Answer from the drawing. Dimensions are ordinates in mm from the lowest x, y and z of the part. A direction names the side the tool comes from. Coordinates: 2 decimals unless noted, no trailing zeros. Loops run counter-clockwise (first coordinate to the right, second up) from the corner with the lowest first, then second, coordinate; pieces in that order, holes last. Notation, with made-up numbers: M -7,-39.5 L 31,-39.5 A27 cw 31,-17.5 Z; hole C 40.25,48.5 d4. An arc over 180 degrees is marked long. Answer as CSV lines item,"result". Start each with the question number.
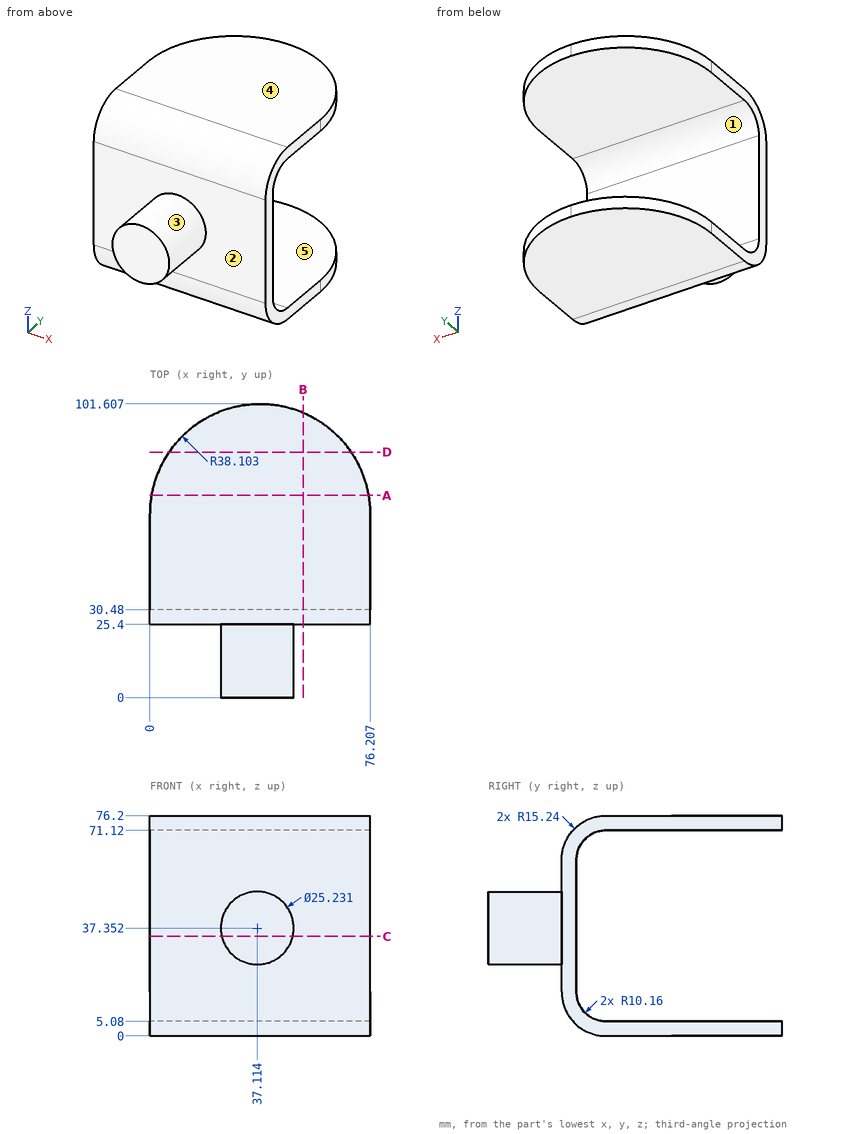
Item 1: Consider line 1 (Z direction, x = 67.5, y = 86); line 2 (Y direction, x = 31, z = 29); line 3 (Y direction, x = 37, z = 23). Determine where each line is inside the solid, lowest interval first.
Item 2: Section D-D on y = 85 is taken. Determine the outline of the cut face in (x, z) (1 decimal).
Item 3: For the marked faces 4 and 5, determine the directions among +Z, -Z, +X, -X, +Y, -Y from which every point of the face is accessible in a straight line to the end or side of a thin tool.
Item 4: Section A-A on y = 70 is taken. Determine the outline of the cut face in (x, z), then the cut area to 3 significant figures.
Item 5: Section C-C on z = 34.5 is taken. Determine the outline of the cut face in (x, y) (1 decimal).
Item 6: Section B-B on x = 53 is taken. Determine the outline of the cut face in (y, z) (1 decimal).
Item 7: Each of these flat-tipped pins is pushed along its axis until it touches: P1, Ø10, axis at x = 35, z = 52, coming from the +Y side; P2, Ø2, axis at x = 13.5, y = 24, coming from the +Z side; P3, Ø3, axis at x = 48.5, y = 37.5, coming from the -Z side; P4, Ø2, axis at x = 33, y = 10.5, coming from the +Z side. Where does it stop, or does it pass through?
Item 8: For a pull along Z with two mould halves and no side action, classify the marked faces 1, 2 and 3 as pulls with the +Z half, pulls with the -Z half, needs draft (parallel to the pull), parting line crosses it, or undercut.
Results are:
1,line 1,"0 to 5.08, 71.12 to 76.2"
1,line 2,"0 to 30.48"
1,line 3,"25.4 to 30.48"
2,outline,"M 6.6,0 L 69.6,0 L 69.6,5.1 L 6.6,5.1 Z; M 6.6,71.1 L 69.6,71.1 L 69.6,76.2 L 6.6,76.2 Z"
3,face 4,"+Z, +X, -X, +Y, -Y"
3,face 5,"+X, -X, +Y"
4,outline,"M 0.56,0 L 75.65,0 L 75.65,5.08 L 0.56,5.08 Z; M 0.56,71.12 L 75.65,71.12 L 75.65,76.2 L 0.56,76.2 Z"
4,area,"763 mm²"
5,outline,"M 0,25.4 L 24.8,25.4 L 24.8,0 L 49.4,0 L 49.4,25.4 L 76.2,25.4 L 76.2,30.5 L 0,30.5 Z"
6,outline,"M 25.4,15.2 A15.2 ccw 40.6,0 L 98.6,0 L 98.6,5.1 L 40.6,5.1 A10.2 cw 30.5,15.2 L 30.5,61 A10.2 cw 40.6,71.1 L 98.6,71.1 L 98.6,76.2 L 40.6,76.2 A15.2 ccw 25.4,61 Z"
7,P1,"y = 30.48"
7,P2,"through"
7,P3,"z = 0.09"
7,P4,"z = 49.58"
8,face 1,"undercut"
8,face 2,"needs draft"
8,face 3,"parting line crosses it"
